from build123d import *

# Parameters (mm, degrees)
SKETCH_1_W          = 65
SKETCH_1_H          = 50
EXTRUDE_1_DEPTH     = 12
SKETCH_2_R          = 2.5
CUT_EXTRUDE_1_DEPTH = 10
CUT_EXTRUDE_2_DEPTH = 12
SKETCH_4_R          = 5
CUT_EXTRUDE_3_DEPTH = 12
SKETCH_5_R          = 2.5
CUT_EXTRUDE_4_DEPTH = 10


with BuildPart() as part:
    # 草图1 → 凸台-拉伸1 (new body)
    with BuildSketch(Plane.XY):
        Rectangle(SKETCH_1_W, SKETCH_1_H)
    extrude(amount=EXTRUDE_1_DEPTH)

    # 草图2 → 切除-拉伸1 (cut)
    with BuildSketch(Plane(origin=(0, -25, 0), x_dir=(-1, 0, 0), z_dir=(0, -1, 0))):
        with Locations(Location((7.5, -6, 0), (0, 0, 90))):
            Circle(SKETCH_2_R)
        with Locations(Location((-7.5, -6, 0), (0, 0, 90))):
            Circle(SKETCH_2_R)
        with Locations(Location((-22.5, -6, 0), (0, 0, 90))):
            Circle(SKETCH_2_R)
    extrude(amount=-CUT_EXTRUDE_1_DEPTH, mode=Mode.SUBTRACT)

    # 草图3 → 切除-拉伸2 (cut)
    with BuildSketch(Plane(origin=(0, 0, 0), x_dir=(-1, 0, 0), z_dir=(0, 0, -1))):
        with BuildLine():
            ThreePointArc((-32.5, -15), (-31.035533906, -11.464466094), (-27.5, -10))
            Line((-27.5, -10), (-16.5, -10))
            ThreePointArc((-16.5, -10), (-3.064971157, -4.435028843), (2.5, 9))
            Line((2.5, 9), (2.5, 10))
            ThreePointArc((2.5, 10), (6.893398271, 20.606601706), (17.499999967, 25))
            Line((17.499999967, 25), (-32.5, 25))
            Line((-32.5, 25), (-32.5, -15))
        make_face()
        with BuildLine():
            Line((32.5, 25), (17.499999967, 25))
            ThreePointArc((17.499999967, 25), (28.106601706, 20.606601729), (32.5, 10))
            Line((32.5, 10), (32.5, 25))
        make_face()
    extrude(amount=-CUT_EXTRUDE_2_DEPTH, mode=Mode.SUBTRACT)

    # 草图4 → 切除-拉伸3 (cut)
    with BuildSketch(Plane(origin=(0, 0, 0), x_dir=(-1, 0, 0), z_dir=(0, 0, -1))):
        with Locations((17.5, 10)):
            Circle(SKETCH_4_R)
    extrude(amount=-CUT_EXTRUDE_3_DEPTH, mode=Mode.SUBTRACT)

    # 草图5 → 切除-拉伸4 (cut)
    with BuildSketch(Plane.ZY.offset(32.5)):
        with Locations((5, -15)):
            Circle(SKETCH_5_R)
    extrude(amount=-CUT_EXTRUDE_4_DEPTH, mode=Mode.SUBTRACT)


solid = part.part
Here's how the part is built. I have some questions about the finished solid (model axes, mm). A direction names the side the tool comes from. Round coordinates to 2 decimals unless told otherwise and drop trailing zeros. Write each loop counter-clockwise with the first axis right and the second up, starting at its lowest first coordinate (ties: lowest second). Pieces come first, ordered by that corner, then holes. Notation, with made-up numbers: (-16, 27.25) -> (-8, 27.25) arc R21 ccw to (-8, 36.25) -> close; hole circle Ø2 at (82, 1). An arc over 180 degrees is marked (long way). One line per item, written item: value.
1) Suppose I cut it at D-D on y = 7. List the corners of the cut face in (x, z) for me, plus the area to 3 significant figures.
Filled sheet:
outline: (-32.5, 0) -> (-21.5, 0) -> (-21.5, 12) -> (-32.5, 12) -> close; (-13.5, 0) -> (-2.39, 0) -> (-2.39, 12) -> (-13.5, 12) -> close
area: 265 mm2
2) I'm going to push flat-ended pins straight in: pin 1 Ø1.1 at (y, z) = (9.5, 7.5) entering from +X; pin 2 Ø2.5 at (x, z) = (-8, 6.5) entering from -Y; pin 3 Ø6.5 at (x, z) = (22.5, 6) entering from +Y. Where does each tip first touch, or does it pass through?
Filled sheet:
pin 1: stops at x = -2.5
pin 2: stops at y = -15
pin 3: stops at y = -10
3) For faces 4 (the face through (22, -10, 6)), 5 (the face through (-22.5, -15, 5)), 6 (the face through (-7, -15, 6)), 7 (the face through (32.5, -20, 6)), which set-ups out of +Z, -Z, +X, -X, +Y, -Y let a thin tool reach every point of the face, with its end or its side?
Filled sheet:
face 4: +Z, -Z, +X, +Y
face 5: -X
face 6: -Y
face 7: +Z, -Z, +X, +Y, -Y
4) Suppose I cut it at C-C on z = 5. List the corners of the cut face in (x, y) for me, plus the area to 3 significant figures.
Filled sheet:
outline: (-32.5, -25) -> (-9.79, -25) -> (-9.79, -15) -> (-5.21, -15) -> (-5.21, -25) -> (5.21, -25) -> (5.21, -15) -> (9.79, -15) -> (9.79, -25) -> (20.21, -25) -> (20.21, -15) -> (24.79, -15) -> (24.79, -25) -> (32.5, -25) -> (32.5, -15) arc R5 ccw to (27.5, -10) -> (16.5, -10) arc R19 cw to (-2.5, 9) -> (-2.5, 10) arc R15 ccw to (-32.5, 10) -> (-32.5, -12.5) -> (-22.5, -12.5) -> (-22.5, -17.5) -> (-32.5, -17.5) -> close; hole circle Ø10 at (-17.5, 10)
area: 1,730 mm2
5) Suppose I cut it at B-B on x = 22.5. List the corners of the cut face in (y, z) for me, plus the area to 3 significant figures.
Filled sheet:
outline: (-25, 0) -> (-10, 0) -> (-10, 12) -> (-25, 12) -> (-25, 8.5) -> (-15, 8.5) -> (-15, 3.5) -> (-25, 3.5) -> close
area: 130 mm2
6) Suppose I cut it at A-A on y = -16.5. List the corners of the cut face in (x, z) for me, plus the area to 3 significant figures.
Filled sheet:
outline: (-32.5, 0) -> (32.5, 0) -> (32.5, 12) -> (-32.5, 12) -> (-32.5, 7) -> (-22.5, 7) -> (-22.5, 3) -> (-32.5, 3) -> close; hole circle Ø5 at (-7.5, 6); hole circle Ø5 at (7.5, 6); hole circle Ø5 at (22.5, 6)
area: 681 mm2
7) If I drill on line 1 (X direction, y = -20, z = 6); line 2 (X direction, y = -16, z = 5.5); line 3 (X direction, y = 13, z = 6.5), over which ranges is the centre line in solid material (lowest first)? Write a range as [from, to].
Filled sheet:
line 1: x = [-32.5, -10], [-5, 5], [10, 20], [25, 32.5]
line 2: x = [-22.5, -9.95], [-5.05, 5.05], [9.95, 20.05], [24.95, 32.5]
line 3: x = [-32.2, -21.5], [-13.5, -2.8]
8) We'd pull the mould along Y, two halves only. Please class faces 1 (the face through (5.28, -20.07, 4.85)), 2 (the face through (-16.849, 14.957, 5.916)), 3 (the face through (0, -25, 6)): released by +Y, released by -Y, zero draft, split by the parting line, or undercut.
Filled sheet:
face 1: zero draft
face 2: undercut
face 3: released by -Y
